Work out the finished part from the listing and answer in its coordinate system (mm). Give positions to 0.01 mm unless a question says otherwise; leave off trailing zeros. Order: outer loops, then holes, each group sorted by start corner. A loop starts at its lowest first (then second) coordinate and runs counter-clockwise, first axis right, second up. Notation, with made-up numbers: M -30,-4.5 L -18,-4.5 A27 cw -18,26.5 Z; hole C -15.75,-29.5 d6. An arc over 180 degrees is marked long. One line per item, written item: value.
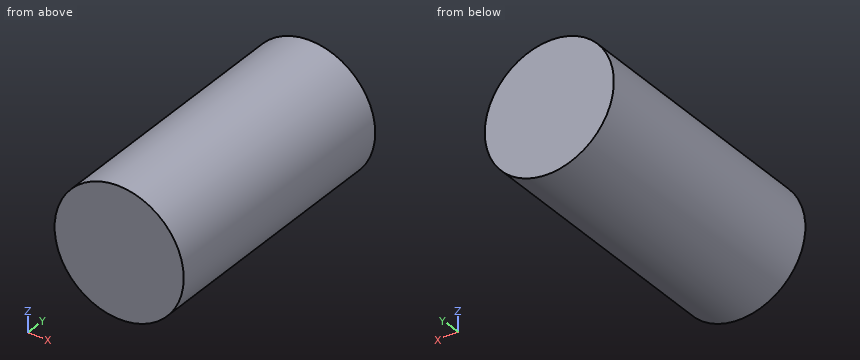
from build123d import *

# Parameters (mm, degrees)
F0_R     = 16.979872
F1_DEPTH = 73
F2_R     = 27.197587
F3_R     = 15.103287
F4_DEPTH = 61.9


with BuildPart() as f1:
    # F0 (on Front) → F1 (new body)
    with BuildSketch(Plane.XZ):
        Polygon((27.902432, 53.963579), (-62.461782, 53.963579), (-43.482464, -46.598472), (49.431205, -19.404227), (30.168617, 24.503149), align=None)
        with Locations((-25.352968, 16.004948)):
            Circle(F0_R, mode=Mode.SUBTRACT)
    extrude(amount=F1_DEPTH)

    # F2
    f2_edges = [f1.edges().sort_by_distance(p)[0] for p in [
        (49.431205, -36.5, -19.404227),
    ]]
    fillet(f2_edges, radius=F2_R)

    # F3 (on face) → F4 (intersect)
    with BuildSketch(Plane.XZ.offset(73)):
        with Locations((11.919588, 11.299165)):
            Circle(F3_R)
    extrude(amount=-F4_DEPTH, mode=Mode.INTERSECT)


solid = f1.part
(1) Section B-B, the plane x = 19 is taken. Give the vertices of the cut face in (y, z), then the cut area to 3 significant figures.
Findings:
outline: M -73,-2.04 L -11.1,-2.04 L -11.1,24.64 L -73,24.64 Z
area: 1,650 mm^2
(2) Given P1, Ø1.5, axis at y = -65, z = 4.5, coming from the -X side; P2, Ø2, axis at x = 0.5, y = -17.5, coming from the -Z side; P3, Ø8, axis at x = 3, y = -57, coming from the +Z side, each flat-ended and moving along its own axis, determine where each tip first touches the part or whether it passes through.
Findings:
P1: stops at x = -1.92
P2: stops at z = 0.37
P3: stops at z = 25.58
(3) Find the intervals of material crossed by probe 1 along Z at (x, y) = (12.5, -37.5); probe 2 along Z at (x, y) = (23, -62.5); probe 3 along X at (y, z) = (-50.5, 20.5), in increasing order. Write a range as from..to.
Findings:
probe 1: z = -3.79..26.39
probe 2: z = 1.04..21.56
probe 3: x = -0.06..23.9
(4) Section C-C, the plane y = -34 is taken. Give the vertices of the cut face in (x, z).
Findings:
outline: C 11.92,11.3 d30.21
(5) Section A-A, the plane z = 0.5 is taken. Give the vertices of the cut face in (x, y), then the cut area to 3 significant figures.
Findings:
outline: M 1.36,-73 L 22.48,-73 L 22.48,-11.1 L 1.36,-11.1 Z
area: 1,310 mm^2
